Build history of the part. All positions in model axes, mm. Face numbers are marked on the shaded views. A direction names the side the tool comes from. Give positions to 0.01 mm unless a question says otherwise; leave off trailing zeros. Order: outer loops, then holes, each group sorted by start corner. A loop starts at its lowest first (then second) coordinate and runs counter-clockwise, first axis right, second up. Notation, with made-up numbers: (32.25, -38) - (70.25, -38) arc R18 ccw to (70.25, -15) - close; hole circle Ø5 at (-18, 18.5). An arc over 180 degrees is marked (long way). One line per item, written item: value.
```python
from build123d import *

# Parameters (mm, degrees)
SKETCH2_W           = 40
SKETCH2_H           = 12.7
BOSS_EXTRUDE1_DEPTH = 6.35
SKETCH3_W           = 27.3
SKETCH3_H           = 6.35
BOSS_EXTRUDE2_DEPTH = 12.7
SKETCH4_W           = 4.9
SKETCH4_H           = 6.35
CUT_EXTRUDE1_DEPTH  = 8.6
SKETCH5_W           = 14.7
SKETCH5_H           = 6.35
BOSS_EXTRUDE3_DEPTH = 30.95


with BuildPart() as part:
    # Sketch2 → Boss-Extrude1 (new body)
    with BuildSketch(Plane.XY):
        Rectangle(SKETCH2_W, SKETCH2_H)
    extrude(amount=BOSS_EXTRUDE1_DEPTH)

    # Sketch3 → Boss-Extrude2 (add)
    with BuildSketch(Plane.XZ.offset(6.35)):
        with Locations((0, 3.175)):
            Rectangle(SKETCH3_W, SKETCH3_H)
    extrude(amount=BOSS_EXTRUDE2_DEPTH)

    # Sketch4 → Cut-Extrude1 (cut)
    with BuildSketch(Plane(origin=(0, 6.35, 0), x_dir=(1, 0, 0), z_dir=(0, 1, 0))):
        with Locations((0, -3.175)):
            Rectangle(SKETCH4_W, SKETCH4_H)
    extrude(amount=-CUT_EXTRUDE1_DEPTH, mode=Mode.SUBTRACT)

    # Sketch5 → Boss-Extrude3 (add)
    with BuildSketch(Plane.XZ.offset(19.05)):
        with Locations((0, 3.175)):
            Rectangle(SKETCH5_W, SKETCH5_H)
    extrude(amount=BOSS_EXTRUDE3_DEPTH)


solid = part.part
```
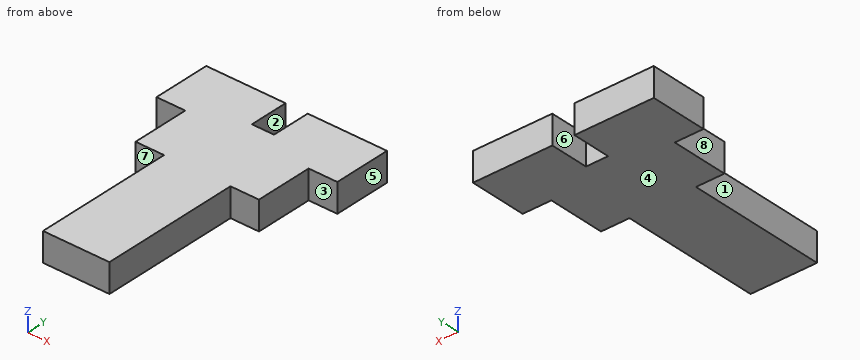
(1) 3-axis set-ups, long thin cutter, end or side, ignore diameter. For the marked faces 1, 2, 3 and 4: which of +Z, -Z, +X, -X, +Y, -Y reach the whole face in a straight line?
Completed:
face 1: +Z, -Z, -X, -Y
face 2: +Z, -Z, +Y
face 3: +Z, -Z, +X, -Y
face 4: -Z, +X, -X, +Y, -Y
(2) Slice it at A-A, the plane z = 5. Give the cut face in (x, y).
Completed:
outline: (-20, -6.35) - (-13.65, -6.35) - (-13.65, -19.05) - (-7.35, -19.05) - (-7.35, -50) - (7.35, -50) - (7.35, -19.05) - (13.65, -19.05) - (13.65, -6.35) - (20, -6.35) - (20, 6.35) - (2.45, 6.35) - (2.45, -2.25) - (-2.45, -2.25) - (-2.45, 6.35) - (-20, 6.35) - close
(3) Pin check, flat tips, straight feed: P1, Ø1.9, axis at x = -10.5, z = 2, coming from the -Y side; P2, Ø2.5, axis at x = -1, z = 3.5, coming from the +Y side; P3, Ø1.9, axis at x = 16, z = 3.5, coming from the -Y side. Stop position of each tip, or through.
Completed:
P1: y = -19.05
P2: y = -2.25
P3: y = -6.35
(4) Slice it at B-B, the plane y = -26.5. Give the cut face in (x, z).
Completed:
outline: (-7.35, 0) - (7.35, 0) - (7.35, 6.35) - (-7.35, 6.35) - close
(5) Drill centre lines: line 1 (X direction, y = -23.5, z = 1.75); line 2 (Y direction, x = -17, z = 0.75); line 3 (X direction, y = 0.5, z = 2.25). Where is each one in solid material? Low to high.
Completed:
line 1: -7.35 to 7.35
line 2: -6.35 to 6.35
line 3: -20 to -2.45, 2.45 to 20
(6) Slice it at C-C, the plane x = -9.5. Give the cut face in (y, z).
Completed:
outline: (-19.05, 0) - (6.35, 0) - (6.35, 6.35) - (-19.05, 6.35) - close
(7) Pull direction X, two halves, no side cores. Call the marked faces 5, 6, 7 and 8: +X half, -X half, draft (parallel to the pull), parting line (faces both ways), or undercut.
Completed:
face 5: +X half
face 6: undercut
face 7: draft
face 8: -X half
